Read the model definition and answer for the solid it produces. Units are mm, in the model's axes. A direction names the side the tool comes from. Coordinates: 2 decimals unless noted, no trailing zeros. Order: outer loops, then holes, each group sorted by start corner. A loop starts at its lowest first (then second) coordinate and runs counter-clockwise, first axis right, second up. Notation, with made-up numbers: (-26, 62) - (22, 62) arc R28 ccw to (22, 81) - close; hole circle Ø8 at (57, -38.75). An arc over 180 degrees is marked (long way). Use one line per item in the form item = value.
```python
from build123d import *

# Parameters (mm, degrees)
BOSS_EXTRUDE1_DEPTH = 3.175
SKETCH2_W           = 63.5
SKETCH2_H           = 6.35
CUT_EXTRUDE1_DEPTH  = 1.5875


with BuildPart() as part:
    # Sketch1 → Boss-Extrude1 (new body)
    with BuildSketch(Plane.XY):
        Polygon((0, 0), (63.5, 0), (63.5, 76.2), (98.679, 76.2), (98.679, 107.95), (63.5, 107.95), (0, 107.95), align=None)
    extrude(amount=BOSS_EXTRUDE1_DEPTH)

    # Sketch2 → Cut-Extrude1 (cut)
    with BuildSketch(Plane.XY.offset(3.175)):
        with Locations((31.75, 3.175)):
            Rectangle(SKETCH2_W, SKETCH2_H)
    extrude(amount=-CUT_EXTRUDE1_DEPTH, mode=Mode.SUBTRACT)


solid = part.part
```
(1) Section C-C, the plane y = 64 is taken. Write down the section's boundary in (x, z) (3 decimals), then the cut area to 3 significant figures.
Answer list:
outline = (0, 0) - (63.5, 0) - (63.5, 3.175) - (0, 3.175) - close
area = 202 mm2
(2) Section B-B, the plane z = 0.95 is taken. Write down the section's boundary in (x, y), then the cut area to 3 significant figures.
Answer list:
outline = (0, 0) - (63.5, 0) - (63.5, 76.2) - (98.68, 76.2) - (98.68, 107.95) - (0, 107.95) - close
area = 7,970 mm2
(3) Which of the six approach directions +Z, -Z, +X, -X, +Y, -Y give full straight-line access (tool end or side, diameter ignored) to faces 1 (the flat face through (31, 3, 1.588)), 2 (the flat face through (0, 55, 2)), 3 (the flat face through (81, 76.2, 2))?
Answer list:
face_1 = +Z, +X, -X, -Y
face_2 = +Z, -Z, -X, +Y, -Y
face_3 = +Z, -Z, +X, -Y
(4) Straight lines are drawn through the part: L1, parallel to X at y = 40, z = 2.7; L2, parallel to Y at x = 15, z = 1.7; L3, parallel to Y at x = 82.5, z = 1.95. For each, find the intervals that lie inside material, in ascending order.
Answer list:
L1 = 0 to 63.5
L2 = 6.35 to 107.95
L3 = 76.2 to 107.95
(5) Given pin 1 Ø0.8 at (x, z) = (46.5, 2.5) entering from -Y; pin 2 Ø1.9 at (x, y) = (31, 4) entering from +Z; pin 3 Ø1 at (x, z) = (88, 2) entering from -Y; pin 4 Ø12 at (x, y) = (57, 32) entering from -Z, each flat-ended and moving along its own axis, determine where each tip first touches the part or whether it passes through.
Answer list:
pin_1 = 6.35
pin_2 = 1.59
pin_3 = 76.2
pin_4 = 0
